Drawing for the job (mm, zero at the part's lowest x, y, z). A direction names the side the tool comes from. Round coordinates to 2 decimals unless told otherwise and drop trailing zeros. Order: outer loops, then holes, each group sorted by start corner. A loop starts at its lowest first (then second) coordinate and runs counter-clockwise, first axis right, second up. Notation, with made-up numbers: (-7, -13.75) -> (19, -13.75) arc R30 ccw to (19, 16.25) -> close; hole circle Ø5 at (19.25, 55). An arc over 180 degrees is marked (long way). Use CSV: the item, a comma, the result in double quotes.
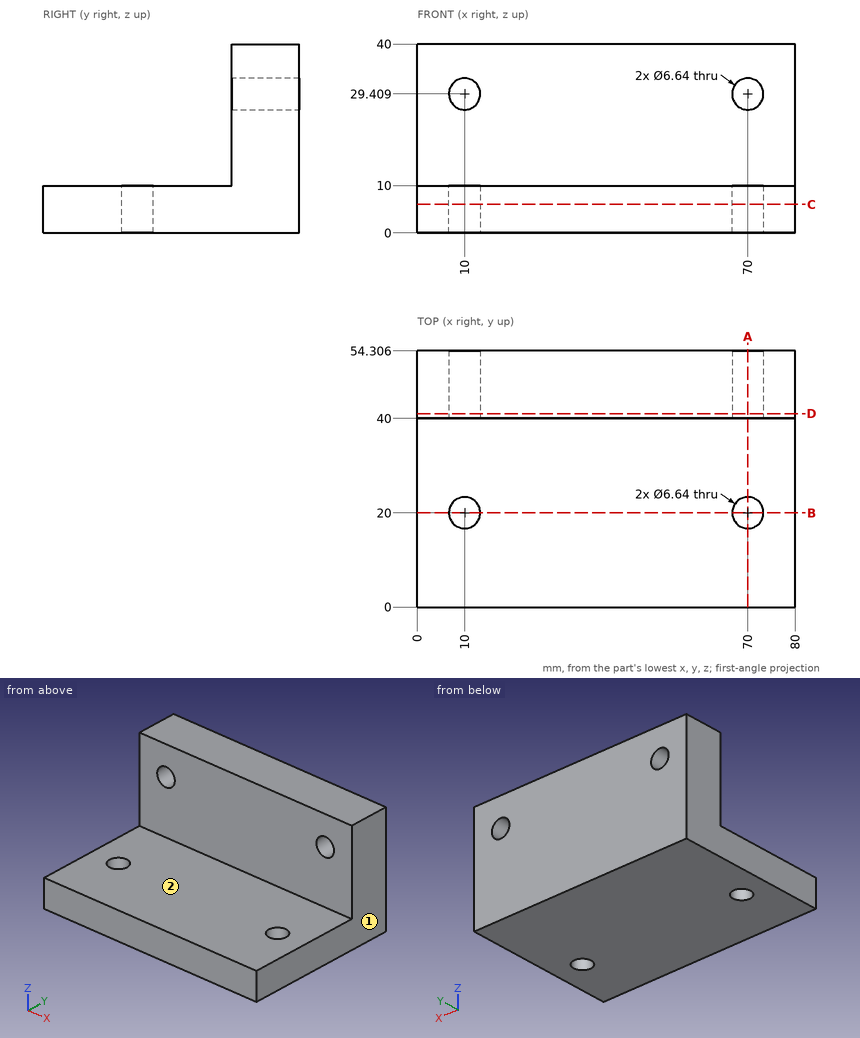
Q1. Cut at B-B (y = 20). Give the cut face in (x, z), plus the area to 3 significant figures.
From the geometry:
outline,"(0, 0) -> (6.68, 0) -> (6.68, 10) -> (0, 10) -> close; (13.32, 0) -> (66.68, 0) -> (66.68, 10) -> (13.32, 10) -> close; (73.32, 0) -> (80, 0) -> (80, 10) -> (73.32, 10) -> close"
area,"667 mm²"
Q2. Pin check, flat tips, straight feed: pin 1 (10 mm diameter, centred on x = 62.5, y = 34.5, fed in from +Z); pin 2 (1.5 mm diameter, centred on x = 42.5, z = 16, fed in from -Y). Stop position of each tip, or through.
From the geometry:
pin 1,"stops at z = 10"
pin 2,"stops at y = 40"
Q3. Cut at A-A (x = 70). Give the cut face in (y, z), plus the area to 3 significant figures.
From the geometry:
outline,"(0, 0) -> (16.68, 0) -> (16.68, 10) -> (0, 10) -> close; (23.32, 0) -> (54.31, 0) -> (54.31, 26.09) -> (40, 26.09) -> (40, 10) -> (23.32, 10) -> close; (40, 32.73) -> (54.31, 32.73) -> (54.31, 40) -> (40, 40) -> close"
area,"811 mm²"
Q4. Probe line 1 along Y through (x, z) = (10, 7); line 2 along X through (y, z) = (18, 4); line 3 along Z through (x, y) = (69.5, 16.5). List the from-to ranges inside material, lowest first.
From the geometry:
line 1,"y = 0 to 16.68, 23.32 to 54.31"
line 2,"x = 0 to 7.35, 12.65 to 67.35, 72.65 to 80"
line 3,"z = 0 to 10"
Q5. Cut at C-C (z = 6). Give the cut face in (x, y).
From the geometry:
outline,"(0, 0) -> (80, 0) -> (80, 54.31) -> (0, 54.31) -> close; hole circle Ø6.64 at (10, 20); hole circle Ø6.64 at (70, 20)"
Q6. Which spindle directions (+Z, -Z, +X, -X, +Y, -Y) get a long thin tool onto all of the face, cutting with end or side? Do the marked faces 1 and 2. Say none if no direction does.
From the geometry:
face 1,"+Z, -Z, +X, +Y, -Y"
face 2,"+Z, +X, -X, -Y"
Q7. Cut at D-D (y = 41). Give the cut face in (x, z), plus the area to 3 significant figures.
From the geometry:
outline,"(0, 0) -> (80, 0) -> (80, 40) -> (0, 40) -> close; hole circle Ø6.64 at (10, 29.41); hole circle Ø6.64 at (70, 29.41)"
area,"3,130 mm²"
